from build123d import *

# Parameters (mm, degrees)
F0_W     = 203.2
F0_H     = 39.6875
F1_DEPTH = 6.35
F3_DEPTH = 6.35
F5_DEPTH = 12.7
F6_W     = 203.2
F6_H     = 7.9375
F7_DEPTH = 3.175
F8_W     = 203.2
F8_H     = 7.9375
F9_DEPTH = 3.175


with BuildPart() as f1:
    # F0 (on Front) → F1 (new body, symmetric)
    with BuildSketch(Plane.XZ):
        Rectangle(F0_W, F0_H)
    extrude(amount=F1_DEPTH, both=True)

    # F2 (on Front) → F3 (join, symmetric)
    with BuildSketch(Plane.XZ):
        with BuildLine():
            Line((107.95, 2.38125), (101.6, 2.38125))
            Line((101.6, 2.38125), (101.6, -3.96875))
            Line((101.6, -3.96875), (107.95, -3.96875))
            ThreePointArc((107.95, -3.96875), (118.0659966007, -0.79375), (107.95, 2.38125))
        make_face()
    extrude(amount=F3_DEPTH, both=True)

    # F4 (on Front) → F5 (cut, symmetric)
    with BuildSketch(Plane.XZ):
        with BuildLine():
            Line((-95.25, 2.38125), (-101.6, 2.38125))
            Line((-101.6, 2.38125), (-101.6, -3.96875))
            Line((-101.6, -3.96875), (-95.25, -3.96875))
            ThreePointArc((-95.25, -3.96875), (-85.1340033993, -0.79375), (-95.25, 2.38125))
        make_face()
    extrude(amount=F5_DEPTH, both=True, mode=Mode.SUBTRACT)

    # F6 (on face) → F7 (cut)
    with BuildSketch(Plane.XZ.offset(6.35)):
        with Locations((0, 11.1125)):
            Rectangle(F6_W, F6_H)
    extrude(amount=-F7_DEPTH, mode=Mode.SUBTRACT)

    # F8 (on face) → F9 (cut)
    with BuildSketch(Plane.XZ.offset(6.35)):
        with Locations((0, -11.1125)):
            Rectangle(F8_W, F8_H)
    extrude(amount=-F9_DEPTH, mode=Mode.SUBTRACT)


solid = f1.part
Build history of the part. All positions in model axes, mm. A direction names the side the tool comes from. Round coordinates to 2 decimals unless told otherwise and drop trailing zeros. Write each loop counter-clockwise with the first axis right and the second up, starting at its lowest first coordinate (ties: lowest second). Pieces come first, ordered by that corner, then holes. Notation, with made-up numbers: M -14,-2 L 18,-2 A6 cw 18,6 Z; hole C 46.25,-15.75 d11. An arc over 180 degrees is marked long. Use CSV: the item, a comma, the result in double quotes.
1. Saw through at B-B (y = -0.75). Give the cut face in (x, z).
Reply:
outline,"M -101.6,-19.84 L 101.6,-19.84 L 101.6,-3.97 L 107.95,-3.97 A5.56 ccw long 107.95,2.38 L 101.6,2.38 L 101.6,19.84 L -101.6,19.84 L -101.6,2.38 L -95.25,2.38 A5.56 cw long -95.25,-3.97 L -101.6,-3.97 Z"
2. Two-plate mould, pull along X, no slides. Class faces 4 (the face through (-101.6, 0, 11)), 5 (the face through (101.6, 0, -12)), 6 (the face through (-1, -6.35, 17)): +X half, -X half, draft (parallel to the pull), parting line (faces both ways), or undercut.
Reply:
face 4,"-X half"
face 5,"undercut"
face 6,"draft"
3. Tool access for faces 1 (the face through (105, 0, -3.969)), 2 (the face through (-1, -3.175, -11)), 3 (the face through (-98, 0, -3.969)): list every direction of +Z, -Z, +X, -X, +Y, -Y with a clear straight run to the whole face (end or side of a thin tool).
Reply:
face 1,"-Z, +Y, -Y"
face 2,"+X, -X, -Y"
face 3,"-X, +Y, -Y"
4. Saw through at C-C (z = 10). Give the cut face in (x, y) (3 decimals).
Reply:
outline,"M -101.6,-3.175 L 101.6,-3.175 L 101.6,6.35 L -101.6,6.35 Z"
5. Wall check: probe 1 along Z at (x, y) = (84.5, -5.5); probe 2 along Y at (x, z) = (23, 8) (3 decimals); probe 3 along X at (y, z) = (2.25, 18). Give the ranges that are in metal, low to high. Write a range as from..to.
Reply:
probe 1,"z = -19.84..-15.08, -7.14..7.14, 15.08..19.84"
probe 2,"y = -3.175..6.35"
probe 3,"x = -101.6..101.6"
6. Flat gauge pins, fed straight in: pin 1 (4 mm diameter, centred on y = -2, z = 8, fed in from +X); pin 2 (5 mm diameter, centred on y = -0.5, z = -6, fed in from +X); pin 3 (2.5 mm diameter, centred on x = -41.5, z = -10, fed in from -Y) (3 decimals). Where does each tip first touch, or does it go through?
Reply:
pin 1,"stops at x = 101.6"
pin 2,"stops at x = 117.36"
pin 3,"stops at y = -3.175"
7. Saw through at A-A (x = 77). Give the cut face in (y, z) (3 decimals).
Reply:
outline,"M -6.35,-19.844 L 6.35,-19.844 L 6.35,19.844 L -6.35,19.844 L -6.35,15.081 L -3.175,15.081 L -3.175,7.144 L -6.35,7.144 L -6.35,-7.144 L -3.175,-7.144 L -3.175,-15.081 L -6.35,-15.081 Z"
8. Saw through at D-D (z = -0.5). Give the cut face in (x, y).
Reply:
outline,"M -85.14,-6.35 L 118.06,-6.35 L 118.06,6.35 L -85.14,6.35 Z"
